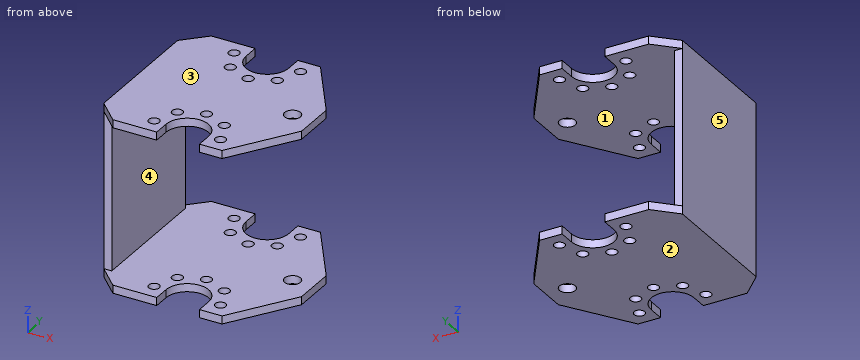
```python
from build123d import *

# Parameters (mm, degrees)
F0_R     = 1
F0_R_2   = 1.5
F1_DEPTH = 1.5
F3_DEPTH = 1.5
F4_W     = 1.5
F4_H     = 24
F5_DEPTH = 14.65


with BuildPart() as f1:
    # F0 (on Top) → F1 (new body)
    with BuildSketch(Plane.XY):
        with BuildLine():
            Line((-4, 16), (-16.22254, 16))
            Line((-16.22254, 16), (-16.22254, -16))
            Line((-16.22254, -16), (-4, -16))
            Line((-4, -16), (-4, -13))
            ThreePointArc((-4, -13), (0, -9), (4, -13))
            Line((4, -13), (4, -16))
            Line((4, -16), (16.22254, -16))
            Line((16.22254, -16), (16.22254, 16))
            Line((16.22254, 16), (4, 16))
            Line((4, 16), (4, 13))
            ThreePointArc((4, 13), (0, 9), (-4, 13))
            Line((-4, 13), (-4, 16))
        make_face()
        with Locations((-6.22254, -13)):
            Circle(F0_R, mode=Mode.SUBTRACT)
        with Locations((-4.4, -8.6)):
            Circle(F0_R, mode=Mode.SUBTRACT)
        with Locations((6.22254, -13)):
            Circle(F0_R, mode=Mode.SUBTRACT)
        with Locations((4.4, -8.6)):
            Circle(F0_R, mode=Mode.SUBTRACT)
        with Locations((0, -6.77746)):
            Circle(F0_R, mode=Mode.SUBTRACT)
        with Locations((-4.4, 8.6)):
            Circle(F0_R, mode=Mode.SUBTRACT)
        with Locations((-6.22254, 13)):
            Circle(F0_R, mode=Mode.SUBTRACT)
        with Locations((0, 6.77746)):
            Circle(F0_R, mode=Mode.SUBTRACT)
        with Locations((12.22254, 0)):
            Circle(F0_R_2, mode=Mode.SUBTRACT)
        with Locations((4.4, 8.6)):
            Circle(F0_R, mode=Mode.SUBTRACT)
        with Locations((6.22254, 13)):
            Circle(F0_R, mode=Mode.SUBTRACT)
    extrude(amount=F1_DEPTH)

    # F2 (on face) → F3 (cut, through all)
    with BuildSketch(Plane.XY.offset(1.5)):
        Polygon((16.22254, 16), (8.22254, 16), (16.22254, 4), align=None)
        Polygon((8.22254, -16), (16.22254, -16), (16.22254, -4), align=None)
        Polygon((-12.22254, 16), (-16.22254, 16), (-16.22254, 12), align=None)
        Polygon((-16.22254, -16), (-12.22254, -16), (-16.22254, -12), align=None)
    extrude(amount=-F3_DEPTH, mode=Mode.SUBTRACT)

    # F4 (on face) → F5 (join)
    with BuildSketch(Plane(origin=(0, 0, 0), x_dir=(1, 0, 0), z_dir=(0, 0, -1))):
        with Locations((-15.47254, 0)):
            Rectangle(F4_W, F4_H)
    extrude(amount=F5_DEPTH)

    # F7: F1 across plane


with BuildPart() as f1_1:
    add(f1.part)
    add(f1.part.mirror(Plane.XY.offset(-14.65)))


solid = f1_1.part
```
Here's how the part is built. I have some questions about the finished solid (model axes, mm). Face numbers are marked on the shaded views. A direction names the side the tool comes from. Round coordinates to 2 decimals unless told otherwise and drop trailing zeros. Loops run counter-clockwise (first coordinate to the right, second up) from the corner with the lowest first, then second, coordinate; pieces in that order, holes last.
1. Suppose I cut it at C-C, the plane x = 10. Please give me the cut outline in (y, z), and give its area (3 significant figures).
Answers:
outline: (-13.33, -30.8) - (13.33, -30.8) - (13.33, -29.3) - (-13.33, -29.3) - close; (-13.33, 0) - (13.33, 0) - (13.33, 1.5) - (-13.33, 1.5) - close
area: 80.0 mm2
2. Suppose I cut it at B-B, the plane y = -13.5. Give the number of separate pieces and of enclosed holes in the cut face, and give its area (3 significant figures).
Answers:
separate pieces: 8
enclosed holes: 0
area: 39.4 mm2
3. Suppose I cut it at D-D, the plane z = -20. Please give me the cut outline in (x, y), and give its area (3 significant figures).
Answers:
outline: (-16.22, -12) - (-14.72, -12) - (-14.72, 12) - (-16.22, 12) - close
area: 36.0 mm2
4. If I drill on probe 1 along Z at (x, y) = (2.5, 5); probe 2 along X at (y, z) = (-10, -25.5); probe 3 along Y at (x, z) = (-15, -29), over which ranges is the centre line in solid material (lowest first)?
Answers:
probe 1: z = -30.8 to -29.3, 0 to 1.5
probe 2: x = -16.22 to -14.72
probe 3: y = -12 to 12
5. For the marked faces 4 and 5, which set-ups out of +Z, -Z, +X, -X, +Y, -Y let a thin tool reach every point of the face, with its end or its side?
Answers:
face 4: +X, +Y, -Y
face 5: +Z, -Z, -X, +Y, -Y
6. Thinking about a two-plate mould opening in Z: for the marked faces 1, 2 and 3, which applies, released by +Z, released by -Z, zero draft, split by the parting line, or undercut?
Answers:
face 1: undercut
face 2: released by -Z
face 3: released by +Z
7. Will these pins go through, and if not, where does the flat tip stop? pin 1 (2.5 mm diameter, centred on x = 12.22, y = 0, fed in from -Z); pin 2 (0.8 mm diameter, centred on x = -15.5, z = -11.5, fed in from -Y); pin 3 (0.8 mm diameter, centred on y = -15, z = -30.5, fed in from -X); pin 4 (1.2 mm diameter, centred on y = 15, z = 1, fed in from +X).
Answers:
pin 1: passes through
pin 2: stops at y = -12
pin 3: stops at x = -13.62
pin 4: stops at x = 9.29
8. Suppose I cut it at A-A, the plane x = 0. Please give me the cut outline in (y, z), and give its area (3 significant figures).
Answers:
outline: (-9, -30.8) - (-7.78, -30.8) - (-7.78, -29.3) - (-9, -29.3) - close; (-9, 0) - (-7.78, 0) - (-7.78, 1.5) - (-9, 1.5) - close; (-5.78, -30.8) - (5.78, -30.8) - (5.78, -29.3) - (-5.78, -29.3) - close; (-5.78, 0) - (5.78, 0) - (5.78, 1.5) - (-5.78, 1.5) - close; (7.78, -30.8) - (9, -30.8) - (9, -29.3) - (7.78, -29.3) - close; (7.78, 0) - (9, 0) - (9, 1.5) - (7.78, 1.5) - close
area: 42.0 mm2
